```python
from build123d import *

# Parameters (mm, degrees)
SKETCH1_R           = 1.25
SKETCH1_W           = 179.84
SKETCH1_H           = 3
SKETCH1_H_2         = 6.62
BOSS_EXTRUDE1_DEPTH = 5
BOSS_EXTRUDE2_START = 5
SKETCH1_3_W         = 179.84
SKETCH1_3_H         = 3
BOSS_EXTRUDE2_DEPTH = 20
FILLET1_R           = 10
FILLET2_R           = 10


with BuildPart() as part:
    # Sketch1 → Boss-Extrude1 (new body)
    # profile 1 of 4: a face of its own
    with BuildSketch(Plane(origin=(0, 0, 0), x_dir=(1, 0, 0), z_dir=(0, 1, 0))):
        with BuildLine():
            Line((98.928888889, 12.527973461), (-80.911111111, 12.527973461))
            Line((-80.911111111, 12.527973461), (-80.911111111, -7.472026539))
            ThreePointArc((-80.911111111, -7.472026539), (-77.982178923, -14.543094351), (-70.911111111, -17.472026539))
            Line((-70.911111111, -17.472026539), (88.928888889, -17.472026539))
            ThreePointArc((88.928888889, -17.472026539), (95.999956701, -14.543094351), (98.928888889, -7.472026539))
            Line((98.928888889, -7.472026539), (98.928888889, 12.527973461))
        make_face()
        with Locations(Location((-75.911111111, -2.972026539, 0), (0, 0, 270))):
            Circle(SKETCH1_R, mode=Mode.SUBTRACT)
        with Locations(Location((-50.911111111, -2.972026539, 0), (0, 0, 270))):
            Circle(SKETCH1_R, mode=Mode.SUBTRACT)
        with Locations(Location((-25.911111111, -2.972026539, 0), (0, 0, 270))):
            Circle(SKETCH1_R, mode=Mode.SUBTRACT)
        with Locations(Location((-0.911111111, -2.972026539, 0), (0, 0, 270))):
            Circle(SKETCH1_R, mode=Mode.SUBTRACT)
        with Locations(Location((18.928888889, -2.972026539, 0), (0, 0, 270))):
            Circle(SKETCH1_R, mode=Mode.SUBTRACT)
        with Locations(Location((43.928888889, -2.972026539, 0), (0, 0, 270))):
            Circle(SKETCH1_R, mode=Mode.SUBTRACT)
        with Locations(Location((68.928888889, -2.972026539, 0), (0, 0, 270))):
            Circle(SKETCH1_R, mode=Mode.SUBTRACT)
        with Locations(Location((93.928888889, -2.972026539, 0), (0, 0, 270))):
            Circle(SKETCH1_R, mode=Mode.SUBTRACT)
    # profile 2 of 4: a face of its own
    with BuildSketch(Plane(origin=(0, 0, 0), x_dir=(1, 0, 0), z_dir=(0, 1, 0))):
        with Locations((9.008888889, 14.027973461)):
            Rectangle(SKETCH1_W, SKETCH1_H)
    # profile 3 of 4: a face of its own
    with BuildSketch(Plane(origin=(0, 0, 0), x_dir=(1, 0, 0), z_dir=(0, 1, 0))):
        with Locations((9.008888889, 18.837973461)):
            Rectangle(SKETCH1_W, SKETCH1_H_2)
    # profile 4 of 4: a face of its own
    with BuildSketch(Plane(origin=(0, 0, 0), x_dir=(1, 0, 0), z_dir=(0, 1, 0))):
        with Locations((9.008888889, 23.647973461)):
            Rectangle(SKETCH1_W, SKETCH1_H)
    extrude(amount=BOSS_EXTRUDE1_DEPTH)

    # Sketch1<3> → Boss-Extrude2 (add)
    with BuildSketch(Plane(origin=(0, 0, 0), x_dir=(1, 0, 0), z_dir=(0, 1, 0)).offset(BOSS_EXTRUDE2_START)):
        with Locations((9.008888889, 14.027973461)):
            Rectangle(SKETCH1_3_W, SKETCH1_3_H)
        with Locations((9.008888889, 23.647973461)):
            Rectangle(SKETCH1_3_W, SKETCH1_3_H)
    extrude(amount=BOSS_EXTRUDE2_DEPTH)

    # Fillet1
    fillet1_edges = [part.edges().sort_by_distance(p)[0] for p in [
        (9.008888889, 5, -12.527973461),
    ]]
    fillet(fillet1_edges, radius=FILLET1_R)

    # Fillet2
    fillet2_edges = [part.edges().sort_by_distance(p)[0] for p in [
        (-80.911111111, 25, -23.647973461),
        (-80.911111111, 25, -14.027973461),
        (98.928888889, 25, -14.027973461),
        (98.928888889, 25, -23.647973461),
    ]]
    fillet(fillet2_edges, radius=FILLET2_R)


solid = part.part
```
Geometry check sheet. Reference: the model listing, model coordinates, mm. A direction names the side the tool comes from. Round coordinates to 2 decimals unless told otherwise and drop trailing zeros. Order: outer loops, then holes, each group sorted by start corner. A loop starts at its lowest first (then second) coordinate and runs counter-clockwise, first axis right, second up. Notation, with made-up numbers: (25, -12) -> (38, -12) arc R25 ccw to (38, 0) -> close; hole circle Ø3 at (-30, -15). An arc over 180 degrees is marked (long way). Return JSON: item names as keys, results as strings. Group by question number.
Q1. Gauge pin test, flat ends, axial feed: pin 1 (1.5 mm diameter, centred on x = 5.5, y = 15.5, fed in from +Z); pin 2 (3 mm diameter, centred on x = 43.93, z = 2.97, fed in from +Y); pin 3 (8 mm diameter, centred on x = 30, y = 16.5, fed in from +Z). Record the tip position at first contact, or that the pin passes through.
Q2. Tool access check on faces 1 (the flat face through (8, 20, -12.528)), 2 (the flat face through (98.929, 4, -12)), 3 (the flat face through (8, 5, -19)). Record the directions out of +Z, -Z, +X, -X, +Y, -Y that give a thin tool (end or side, any length) a straight path to the whole face; none if there is none.
Q3. Section check C-C, the plane z = -8. Record the boundary of the cut face in (x, y).
Q4. Material ranges on probe 1 along Z at (x, y) = (57.5, 23); probe 2 along Y at (x, z) = (82, 10); probe 3 along Z at (x, y) = (40.5, 8.75), recorded low to high. Write a range as from..to.
Q5. Section check B-B, the plane x = 64.5. Record the boundary of the cut face in (y, z), plus the area to 3 significant figures.
Q6. Section check A-A, the plane y = 7.25. Record the boundary of the cut face in (x, z).
Q7. Release check for a two-part mould opening along Z. For faces 4 (the flat face through (8, 25, -14)), 5 (the flat face through (8, 2, 17.472)), 6 (the flat face through (8, 15, -22.148)) record: released by +Z, released by -Z, zero draft, split by the parting line, or undercut.
Q8. Section check D-D, the plane y = 20.5. Record the boundary of the cut face in (x, z).
Numbers:
{
 "1": {"pin 1": "z = -12.52", "pin 2": "y = 5", "pin 3": "z = -12.21"},
 "2": {"face 1": "+Z, +X, -X, +Y", "face 2": "+Z, -Z, +X, +Y, -Y", "face 3": "+X, -X, +Y"},
 "3": {"outline": "(-80.91, 0) -> (98.93, 0) -> (98.93, 6.63) -> (-80.91, 6.63) -> close"},
 "4": {"probe 1": "-25.15..-22.15, -15.53..-12.53", "probe 2": "0..5", "probe 3": "-25.15..-22.15, -15.53..-10.33"},
 "5": {"outline": "(0, -25.15) -> (25, -25.15) -> (25, -22.15) -> (5, -22.15) -> (5, -15.53) -> (25, -15.53) -> (25, -12.53) -> (15, -12.53) arc R10 cw to (5, -2.53) -> (5, 17.47) -> (0, 17.47) -> close", "area": "355 mm^2"},
 "6": {"outline": "(-80.91, -25.15) -> (98.93, -25.15) -> (98.93, -22.15) -> (-80.91, -22.15) -> close; (-80.91, -15.53) -> (98.93, -15.53) -> (98.93, -8.85) -> (-80.91, -8.85) -> close"},
 "7": {"face 4": "zero draft", "face 5": "released by +Z", "face 6": "undercut"},
 "8": {"outline": "(-79.26, -25.15) -> (97.28, -25.15) -> (97.28, -22.15) -> (-79.26, -22.15) -> close; (-79.26, -15.53) -> (97.28, -15.53) -> (97.28, -12.53) -> (-79.26, -12.53) -> close"}
}
